from build123d import *

# Parameters (mm, degrees)
SKETCH_1_R          = 22.5
EXTRUDE_1_DEPTH     = 4
SKETCH_2_R          = 10
EXTRUDE_2_DEPTH     = 16
FILLET_1_R          = 10
SKETCH_3_R          = 2
CUT_EXTRUDE_1_DEPTH = 10
SKETCH_4_W          = 1
SKETCH_4_H          = 0.5


with BuildPart() as part:
    # Sketch 1 → Extrude 1 (new body)
    with BuildSketch(Plane(origin=(0, 0, 0), x_dir=(1, 0, 0), z_dir=(0, 1, 0))):
        with Locations(Location((0, 0, 0), (0, 0, 270))):
            Circle(SKETCH_1_R)
    extrude(amount=EXTRUDE_1_DEPTH)

    # Sketch 2 → Extrude 2 (add)
    with BuildSketch(Plane(origin=(0, 4, 0), x_dir=(1, 0, 0), z_dir=(0, 1, 0))):
        with Locations(Location((0, 0, 0), (0, 0, 270))):
            Circle(SKETCH_2_R)
    extrude(amount=EXTRUDE_2_DEPTH)

    # Fillet 1
    fillet_1_edges = [part.edges().sort_by_distance(p)[0] for p in [
        (0, 20, -10),
    ]]
    fillet(fillet_1_edges, radius=FILLET_1_R)

    # Sketch 3 → Cut-Extrude 1 (cut)
    with BuildSketch(Plane.XZ):
        with Locations(Location((-13.113453203, 13.401486674, 0), (0, 0, 270))):
            Circle(SKETCH_3_R)
        with Locations(Location((-13.401486674, -13.113453203, 0), (0, 0, 270))):
            Circle(SKETCH_3_R)
        with Locations(Location((13.113453203, -13.401486674, 0), (0, 0, 270))):
            Circle(SKETCH_3_R)
        with Locations(Location((13.401486674, 13.113453203, 0), (0, 0, 270))):
            Circle(SKETCH_3_R)
    extrude(amount=-CUT_EXTRUDE_1_DEPTH, mode=Mode.SUBTRACT)

    # Sketch 4 → Cut-Revolve 1 (revolve, cut)
    with BuildSketch(Plane.XY, mode=Mode.PRIVATE) as cut_revolve_1_sk:
        with Locations((-9.5, 4.25)):
            Rectangle(SKETCH_4_W, SKETCH_4_H)
        with Locations((-9.5, 5.75)):
            Rectangle(SKETCH_4_W, SKETCH_4_H)
        with Locations((-9.5, 7.25)):
            Rectangle(SKETCH_4_W, SKETCH_4_H)
        with Locations((-9.5, 8.75)):
            Rectangle(SKETCH_4_W, SKETCH_4_H)
        with Locations((-9.5, 10.25)):
            Rectangle(SKETCH_4_W, SKETCH_4_H)
        with Locations((-9.5, 11.75)):
            Rectangle(SKETCH_4_W, SKETCH_4_H)
        with Locations((-9.5, 13.25)):
            Rectangle(SKETCH_4_W, SKETCH_4_H)
        with Locations((-9.5, 14.75)):
            Rectangle(SKETCH_4_W, SKETCH_4_H)
        with Locations((-9.5, 16.25)):
            Rectangle(SKETCH_4_W, SKETCH_4_H)
        with Locations((-9.5, 17.75)):
            Rectangle(SKETCH_4_W, SKETCH_4_H)
        with Locations((-9.5, 19.25)):
            Rectangle(SKETCH_4_W, SKETCH_4_H)
    revolve(cut_revolve_1_sk.sketch.rotate(Axis((0, 0, 0), (0, 1, 0)), 270), axis=Axis((0, 0, 0), (0, 1, 0)), mode=Mode.SUBTRACT)


solid = part.part
Source: CAD feature listing. Evaluate the final solid. Frame: model axes, mm. A direction names the side the tool comes from. Round coordinates to 2 decimals unless told otherwise and drop trailing zeros. Loops run counter-clockwise (first coordinate to the right, second up) from the corner with the lowest first, then second, coordinate; pieces in that order, holes last.
Q1. Section A-A, the plane y = 2. Return loops of the section in (x, z), plus the area to 3 significant figures.
Q2. First-contact query: P1, Ø1.5, axis at x = 3.5, z = 2, coming from the -Y side; P2, Ø1, axis at y = 17.5, z = -5.5, coming from the -X side; P3, Ø4, axis at y = 7.5, z = 8.5, coming from the +X side; P4, Ø2, axis at x = -14, z = -6.5, coming from the +Y side. Flat tips, straight axial feed; report the tip coordinate or a pass-through.
Q3. Mould query, pull axis X, two halves, no side actions, for faces 1 (the face through (-12.513, 1.972, 11.494)), 2 (the face through (-2, 5.5, 9)), 3 (the face through (-2.703, 7.254, -8.584)). Classes: pulls with the +X half, pulls with the -X half, needs draft (parallel to the pull), parting line crosses it, or undercut.
Q4. Access query for faces 4 (the face through (13.201, 1.972, -11.403)), 5 (the face through (9, 12, -3)), 6 (the face through (-9.76, 6.49, -2.17)). Directions: +Z, -Z, +X, -X, +Y, -Y. A direction counts if a zero-diameter tool reaches every point of the face in a straight line with its end or side. Return the directions, or none.
Q5. Section C-C, the plane y = 16.5. Return loops of the section in (x, z).
Q6. Section B-B, the plane x = -17. Return loops of the section in (y, z).
Q7. Ray query, line 1 (X direction, y = 3.5, z = 13.5); line 2 (Y direction, x = 0, z = 0.5); line 3 (Y direction, x = 15, z = 8). Return the intervals inside material, ascending.
Solutions:
1. outline: circle Ø45 at (0, 0); hole circle Ø4 at (-13.4, -13.11); hole circle Ø4 at (-13.11, 13.4); hole circle Ø4 at (13.11, -13.4); hole circle Ø4 at (13.4, 13.11)
1. area: 1,540 mm2
2. P1: stops at y = 0
2. P2: stops at x = -4.75
2. P3: stops at x = 7.6
2. P4: stops at y = 4
3. face 1: undercut
3. face 2: needs draft
3. face 3: parting line crosses it
4. face 4: +Y, -Y
4. face 5: none
4. face 6: +Y
5. outline: circle Ø15.2 at (0, 0)
6. outline: (0, -14.74) - (4, -14.74) - (4, 14.74) - (0, 14.74) - close
7. line 1: x = -18 to -15.11, -11.12 to 11.44, 15.36 to 18
7. line 2: y = 0 to 19.99
7. line 3: y = 0 to 4
